```python
from build123d import *

# Parameters (mm, degrees)
BOSS_EXTRUDE1_DEPTH = 10
CUT_EXTRUDE1_REACH  = 126.909
FILLET1_R           = 3
SKETCH3_R           = 1.6
CUT_EXTRUDE2_DEPTH  = 6
SKETCH4_R           = 1.6
CUT_EXTRUDE3_DEPTH  = 7
BOSS_EXTRUDE2_DEPTH = 5
FILLET2_R           = 3
FILLET3_R           = 2
FILLET4_R           = 5
FILLET5_R           = 3
SKETCH7_W           = 25
SKETCH7_H           = 57
BOSS_EXTRUDE3_DEPTH = 7
SKETCH8_R           = 1.304654563
SKETCH8_W           = 21.294220064
SKETCH8_H           = 41
CUT_EXTRUDE4_DEPTH  = 7
FILLET6_R           = 3


with BuildPart() as part:
    # Sketch1 → Boss-Extrude1 (new body)
    with BuildSketch(Plane.XY):
        with BuildLine():
            Line((-13, -85.907758216), (-8, -85.907758216))
            Line((-8, -85.907758216), (-8, -68.093529717))
            Line((-8, -68.093529717), (-20, -68.093529717))
            Line((-20, -68.093529717), (-20, -56.093529717))
            Line((-20, -56.093529717), (20, -56.093529717))
            Line((20, -56.093529717), (20, -68.093529717))
            Line((20, -68.093529717), (8, -68.093529717))
            Line((8, -68.093529717), (8, -85.907758216))
            Line((8, -85.907758216), (13, -85.907758216))
            ThreePointArc((13, -85.907758216), (15.121320344, -86.786437873), (16, -88.907758216))
            Line((16, -88.907758216), (16, -114.907758216))
            ThreePointArc((16, -114.907758216), (15.121320344, -117.02907856), (13, -117.907758216))
            Line((13, -117.907758216), (-13, -117.907758216))
            ThreePointArc((-13, -117.907758216), (-15.121320344, -117.02907856), (-16, -114.907758216))
            Line((-16, -114.907758216), (-16, -88.907758216))
            ThreePointArc((-16, -88.907758216), (-15.121320344, -86.786437873), (-13, -85.907758216))
        make_face()
    extrude(amount=BOSS_EXTRUDE1_DEPTH)

    # Cut-Extrude1: up to this face of the body (flat: up to its plane)
    cut_extrude1_end = Plane(part.part.faces().sort_by_distance((-20, -62.093529717, 5))[0])
    # Sketch2 → Cut-Extrude1 (cut, up to the picked face)
    with BuildSketch(Plane(origin=(20, 0, 0), x_dir=(0, 0, -1), z_dir=(1, 0, 0)), mode=Mode.PRIVATE) as cut_extrude1_sk1:
        with BuildLine():
            Line((-4, -56.093529717), (-4, -75.944087362))
            ThreePointArc((-4, -75.944087362), (-2.946090025, -80.483178975), (0, -84.093529717))
            Line((0, -84.093529717), (0, -56.093529717))
            Line((0, -56.093529717), (-4, -56.093529717))
        make_face()
    cut_extrude1_tool1 = split(extrude(cut_extrude1_sk1.sketch, amount=-CUT_EXTRUDE1_REACH, mode=Mode.PRIVATE), bisect_by=cut_extrude1_end, keep=Keep.BOTH, mode=Mode.PRIVATE)
    add(cut_extrude1_tool1.solids().sort_by(Axis((20, -68.93128, 1.917617), (-1, 0, 0)))[0], mode=Mode.SUBTRACT)

    # Fillet1
    # the kernel refuses this fillet: 3 mm, written as the material it adds along each edge
    with BuildSketch(Plane(origin=(-8, -68.093529717, 4), x_dir=(0, -1, 0), z_dir=(0, 0, 1))) as fillet1_piece_1:
        with BuildLine():
            CenterArc((FILLET1_R, -FILLET1_R), FILLET1_R, 90, 90)
            Line((0, -FILLET1_R), (0, 0))
            Line((0, 0), (FILLET1_R, 0))
        make_face()
    extrude(amount=6)
    with BuildSketch(Plane(origin=(8, -68.093529717, 4), x_dir=(0, -1, 0), z_dir=(0, 0, 1))) as fillet1_piece_2:
        with BuildLine():
            CenterArc((FILLET1_R, FILLET1_R), FILLET1_R, 180, 90)
            Line((0, FILLET1_R), (0, 0))
            Line((0, 0), (FILLET1_R, 0))
        make_face()
    extrude(amount=6)
    with BuildSketch(Plane(origin=(-8, -85.907758216, 0), x_dir=(-1, 0, 0), z_dir=(0, 0, 1))) as fillet1_piece_3_section:
        with BuildLine():
            CenterArc((FILLET1_R, -FILLET1_R), FILLET1_R, 90, 90)
            Line((0, -FILLET1_R), (0, 0))
            Line((0, 0), (FILLET1_R, 0))
        make_face()
    fillet1_piece_3 = extrude(amount=10, mode=Mode.PRIVATE)
    fillet1_piece_3 = fillet1_piece_3 - Plane(origin=(-8.681614659, -75.944087362, -6.301676338), x_dir=(0, 0, 1), z_dir=(1, 0, 0)) * Cylinder(10.301676338, 32, mode=Mode.PRIVATE)
    add(fillet1_piece_3)
    with BuildSketch(Plane(origin=(8, -85.907758216, 0), x_dir=(1, 0, 0), z_dir=(0, 0, 1))) as fillet1_piece_4_section:
        with BuildLine():
            CenterArc((FILLET1_R, FILLET1_R), FILLET1_R, 180, 90)
            Line((0, FILLET1_R), (0, 0))
            Line((0, 0), (FILLET1_R, 0))
        make_face()
    fillet1_piece_4 = extrude(amount=10, mode=Mode.PRIVATE)
    fillet1_piece_4 = fillet1_piece_4 - Plane(origin=(8.68161466, -75.944087362, -6.301676338), x_dir=(0, 0, 1), z_dir=(1, 0, 0)) * Cylinder(10.301676338, 32, mode=Mode.PRIVATE)
    add(fillet1_piece_4)
    # the kernel refuses this fillet: 3 mm, written as the material it takes off along each edge
    with BuildSketch(Plane(origin=(-20, -68.093529717, -3.5), x_dir=(0, 1, 0), z_dir=(0, 0, 1)), Plane(origin=(-20, -56.093529717, -3.5), x_dir=(1, 0, 0), z_dir=(0, 0, 1)), Plane(origin=(20, -56.093529717, -3.5), x_dir=(0, -1, 0), z_dir=(0, 0, 1)), Plane(origin=(20, -68.093529717, -3.5), x_dir=(-1, 0, 0), z_dir=(0, 0, 1))) as fillet1_2_piece_1:
        with BuildLine():
            CenterArc((FILLET1_R, -FILLET1_R), FILLET1_R, 90, 90)
            Line((0, -FILLET1_R), (0, 0))
            Line((0, 0), (FILLET1_R, 0))
        make_face()
    extrude(amount=21, mode=Mode.SUBTRACT)

    # Sketch3 → Cut-Extrude2 (cut)
    with BuildSketch(Plane(origin=(0, 0, 4), x_dir=(-1, 0, 0), z_dir=(0, 0, -1))):
        with Locations(Location((-12, -60.093529717, 0), (0, 0, 90))):
            Circle(SKETCH3_R)
        with Locations(Location((0, -64.093529717, 0), (0, 0, 90))):
            Circle(SKETCH3_R)
        with Locations((12, -60.093529717)):
            Circle(SKETCH3_R)
    extrude(amount=-CUT_EXTRUDE2_DEPTH, mode=Mode.SUBTRACT)

    # Sketch4 → Cut-Extrude3 (cut)
    with BuildSketch(Plane(origin=(0, 0, 0), x_dir=(-1, 0, 0), z_dir=(0, 0, -1))):
        with Locations((11.66726189, -90.240496327)):
            Circle(SKETCH4_R)
        with Locations((-11.66726189, -90.240496327)):
            Circle(SKETCH4_R)
        with Locations((-11.66726189, -113.575020106)):
            Circle(SKETCH4_R)
        with Locations((11.66726189, -113.575020106)):
            Circle(SKETCH4_R)
    extrude(amount=-CUT_EXTRUDE3_DEPTH, mode=Mode.SUBTRACT)

    # Sketch5 → Boss-Extrude2 (add, symmetric)
    with BuildSketch(Plane(origin=(0, 0, 0), x_dir=(0, 0, -1), z_dir=(1, 0, 0))):
        Polygon((-10, -59.093529717), (-10, -54.093529717), (8, -54.093529717), (8, -35.093529717), (88, -35.093529717), (88, -42.093529717), (22, -42.093529717), (14, -49.093529717), (14, -59.093529717), align=None)
    extrude(amount=BOSS_EXTRUDE2_DEPTH, both=True)

    # Fillet2
    # the kernel refuses this fillet: 3 mm, written as the material it adds along each edge
    with BuildSketch(Plane(origin=(-5, -56.093529717, 4), x_dir=(-1, 0, 0), z_dir=(0, 0, 1))) as fillet2_piece_1:
        with BuildLine():
            CenterArc((2.828427125, -3), FILLET2_R, 90, 70.528779366)
            Line((0, -2), (-0.056568542, -1.98))
            ThreePointArc((-0.056568542, -1.98), (-0.06, -1), (-0.06, 0))
            Line((-0.06, 0), (0, 0.06))
            Line((0, 0.06), (2.828427125, 0.06))
            Line((2.828427125, 0.06), (2.828427125, 0))
        make_face()
    extrude(amount=6)
    with BuildSketch(Plane(origin=(5, -56.093529717, 4), x_dir=(1, 0, 0), z_dir=(0, 0, 1))) as fillet2_piece_2:
        with BuildLine():
            CenterArc((2.828427125, 3), FILLET2_R, 199.471220634, 70.528779366)
            Line((0, 2), (-0.056568542, 1.98))
            ThreePointArc((-0.056568542, 1.98), (-0.06, 1), (-0.06, 0))
            Line((-0.06, 0), (0, -0.06))
            Line((0, -0.06), (2.828427125, -0.06))
            Line((2.828427125, -0.06), (2.828427125, 0))
        make_face()
    extrude(amount=6)

    # Fillet3
    fillet3_edges = [part.edges().sort_by_distance(p)[0] for p in [
        (0, -59.093529717, 4),
    ]]
    fillet(fillet3_edges, radius=FILLET3_R)

    # Fillet4
    fillet4_edges = [part.edges().sort_by_distance(p)[0] for p in [
        (0, -59.093529717, -14),
        (0, -54.093529717, -8),
    ]]
    fillet(fillet4_edges, radius=FILLET4_R)

    # Fillet5
    fillet5_edges = [part.edges().sort_by_distance(p)[0] for p in [
        (0, -35.093529717, -8),
    ]]
    fillet(fillet5_edges, radius=FILLET5_R)

    # Sketch7 → Boss-Extrude3 (add)
    with BuildSketch(Plane(origin=(0, -35.093529717, 0), x_dir=(1, 0, 0), z_dir=(0, 1, 0))):
        with Locations((-2.5, 59.5)):
            Rectangle(SKETCH7_W, SKETCH7_H)
    extrude(amount=-BOSS_EXTRUDE3_DEPTH)

    # Sketch8 → Cut-Extrude4 (cut)
    with BuildSketch(Plane(origin=(0, -35.093529717, 0), x_dir=(1, 0, 0), z_dir=(0, 1, 0))):
        with Locations(Location((-4.9, 85.08, 0), (0, 0, 270))):
            Circle(SKETCH8_R)
        with Locations(Location((4.9, 85.08, 0), (0, 0, 270))):
            Circle(SKETCH8_R)
        with Locations(Location((4.9, 36.48, 0), (0, 0, 270))):
            Circle(SKETCH8_R)
        with Locations(Location((-4.9, 36.48, 0), (0, 0, 270))):
            Circle(SKETCH8_R)
        with Locations((0.147110032, 60.78)):
            Rectangle(SKETCH8_W, SKETCH8_H)
    extrude(amount=-CUT_EXTRUDE4_DEPTH, mode=Mode.SUBTRACT)

    # Fillet6
    fillet6_edges = [part.edges().sort_by_distance(p)[0] for p in [
        (0, -49.093529717, -14),
        (0, -42.093529717, -22),
        (5, -38.593529717, -31),
        (-5, -38.593529717, -31),
        (-15, -38.593529717, -31),
        (-15, -38.593529717, -88),
    ]]
    fillet(fillet6_edges, radius=FILLET6_R)


solid = part.part
```
Read the model definition and answer for the solid it produces. Units are mm, in the model's axes. A direction names the side the tool comes from. Give positions to 0.01 mm unless a question says otherwise; leave off trailing zeros. Loops run counter-clockwise (first coordinate to the right, second up) from the corner with the lowest first, then second, coordinate; pieces in that order, holes last.
Item 1: The part is cut by section B-B (y = -93). Write down the section's boundary in (x, z), and give its area (3 significant figures).
Item 2: The part is cut by section A-A (z = -36.48). Write down the section's boundary in (x, y), and give its area (3 significant figures).
Item 3: Each of these flat-tipped pins is pushed along its axis until it touches: pin 1 Ø1.2 at (x, y) = (-10, -39) entering from +Z; pin 2 Ø1 at (x, y) = (-2, -64.5) entering from -Z; pin 3 Ø10 at (y, z) = (-89.5, -9.5) entering from -X; pin 4 Ø1.8 at (x, z) = (-15.5, 5.5) entering from -Y. Where does it stop, or does it pass through?
Item 4: The part is cut by section C-C (z = -56.5). Write down the section's boundary in (x, y), and give its area (3 significant figures).
Item 5: Find the intervals of material crossed by line 1 along Z through (x, y) = (-8, -42); line 2 along Y through (x, z) = (-12, -77); line 3 along Z through (x, y) = (7.5, -109.5), in increasing order.
Item 6: For faces 4 (the cylindrical face through (8.9, -68.95, 6.96)), 5 (the cylindrical face through (10.93, -91.66, 3.45)), 6 (the flat face through (-14, -68.094, 7)), determine the directions among +Z, -Z, +X, -X, +Y, -Y from which every point of the face is accessible in a straight line to the end or side of a thin tool.
Item 7: The mould has two halves that part along Z. Classify faces 1 (the cylindrical face through (19.098, -67.238, 6.958)), 2 (the cylindrical face through (4.957, -38.545, -86.383)), 3 (the flat face through (-1, -39, -88)): released by +Z, released by -Z, zero draft, split by the parting line, or undercut.
Taken from the geometry:
1. outline: (-16, 0) - (16, 0) - (16, 10) - (-16, 10) - close
1. area: 320 mm2
2. outline: (-15, -42.09) - (-6.2, -42.09) - (-6.2, -35.09) - (-15, -35.09) - close; (-3.6, -42.09) - (3.6, -42.09) - (3.6, -35.09) - (-3.6, -35.09) - close; (6.2, -42.09) - (10, -42.09) - (10, -35.09) - (6.2, -35.09) - close
2. area: 138 mm2
3. pin 1: stops at z = -31
3. pin 2: stops at z = 4
3. pin 3: passes through
3. pin 4: stops at y = -117.45
4. outline: (-15, -42.09) - (-10.5, -42.09) - (-10.5, -35.09) - (-15, -35.09) - close
4. area: 31.5 mm2
5. line 1: z = -88 to -81.28, -40.28 to -31
5. line 2: y = -42.09 to -35.09
5. line 3: z = 0 to 10
6. face 4: +Z, -Z, +X
6. face 5: -Z
6. face 6: +Z, -Z, -X
7. face 1: zero draft
7. face 2: undercut
7. face 3: released by -Z
